from build123d import *

# Parameters (mm, degrees)
F0_W     = 17.78
F0_H     = 3.81
F0_W_2   = 3.81
F1_DEPTH = 1.905
F2_DEPTH = 0.9525


with BuildPart() as f1:
    # F0 (on Front) → F1 (new body, symmetric)
    with BuildSketch(Plane.XZ):
        Rectangle(F0_W, F0_H)
        with Locations((10.795, 0)):
            Rectangle(F0_W_2, F0_H)
        with Locations((-10.795, 0)):
            Rectangle(F0_W_2, F0_H)
    extrude(amount=F1_DEPTH, both=True)

    # F0 (on Front) → F2 (join, symmetric)
    with BuildSketch(Plane.XZ):
        with Locations((0, -3.81)):
            Rectangle(F0_W, F0_H)
    extrude(amount=F2_DEPTH, both=True)


solid = f1.part
Could you check a few things on this model? Use its own coordinates, in mm. A direction names the side the tool comes from. Coordinates: 2 decimals unless noted, no trailing zeros. Order: outer loops, then holes, each group sorted by start corner. A loop starts at its lowest first (then second) coordinate and runs counter-clockwise, first axis right, second up. Notation, with made-up numbers: (89, 59) -> (144, 59) arc R15 ccw to (144, 70) -> close; hole circle Ø11 at (-28, -29.5). An arc over 180 degrees is marked (long way). One line per question, with ' | ' between items.
Q1. Imagine slicing it at D-D on x = 9.75. Please give me the cut outline in (y, z) (3 decimals).
Return value:
outline: (-1.905, -1.905) -> (1.905, -1.905) -> (1.905, 1.905) -> (-1.905, 1.905) -> close
Q2. Imagine slicing it at B-B on x = -1. Please give me the cut outline in (y, z) (1 decimal).
Return value:
outline: (-1.9, -1.9) -> (-1, -1.9) -> (-1, -5.7) -> (1, -5.7) -> (1, -1.9) -> (1.9, -1.9) -> (1.9, 1.9) -> (-1.9, 1.9) -> close
Q3. Imagine slicing it at A-A on y = 0.2. Please give me the cut outline in (x, z) (3 decimals).
Return value:
outline: (-12.7, -1.905) -> (-8.89, -1.905) -> (-8.89, -5.715) -> (8.89, -5.715) -> (8.89, -1.905) -> (12.7, -1.905) -> (12.7, 1.905) -> (-12.7, 1.905) -> close
Q4. If I drill on L1, parallel to Y at x = 0.75, z = -5.5; L2, parallel to X at y = 0, z = -3.5; L3, parallel to Z at x = -6.5, y = -1.7 (3 decimals), over which ranges is the centre line in solid material (lowest first)?
Return value:
L1: -0.95 to 0.95 | L2: -8.89 to 8.89 | L3: -1.905 to 1.905
Q5. Imagine slicing it at C-C on z = -3. Please give me the cut outline in (x, y).
Return value:
outline: (-8.89, -0.95) -> (8.89, -0.95) -> (8.89, 0.95) -> (-8.89, 0.95) -> close
Q6. I'm going to push flat-ended pins straight in: P1, Ø1.9, axis at x = -2, z = -3, coming from the -Y side; P2, Ø1, axis at y = 0.5, z = -3.5, coming from the -X side; P3, Ø1.5, axis at x = -9, z = -3.5, coming from the +Y side. Where does each tip first touch, or does it pass through?
Return value:
P1: y = -0.95 | P2: x = -8.89 | P3: y = 0.95
Q7. On a 3-axis mill with a long thin cutter (end or side, diameter ignored), from which of +Z, -Z, +X, -X, +Y, -Y can I reach the whole of each face in a straight line? I mean faces 1 (the face through (0, 0.952, -4)), 2 (the face through (-12.7, 0, 0)), 3 (the face through (-8.89, 0, -4)), 4 (the face through (8.89, 0, -4)), 5 (the face through (0, -0.952, -4)). Say none if no direction works.
Return value:
face 1: -Z, +X, -X, +Y | face 2: +Z, -Z, -X, +Y, -Y | face 3: -Z, -X, +Y, -Y | face 4: -Z, +X, +Y, -Y | face 5: -Z, +X, -X, -Y
